from build123d import *

# Parameters (mm, degrees)
BOSS_EXTRUDE1_DEPTH     = 40
CUT_EXTRUDE1_DEPTH      = 60
SKETCH3_W               = 113.025821482
SKETCH3_H               = 33
CUT_EXTRUDE2_DEPTH      = 25
CUT_EXTRUDE6_DEPTH      = 96.088865234
CUT_EXTRUDE6_DEPTH_BACK = 96.088865234
SKETCH7_W               = 50
SKETCH7_H               = 33
SKETCH8_W               = 71.47426929
SKETCH8_H               = 40
BOSS_EXTRUDE2_DEPTH     = 5
FILLET1_R               = 5
FILLET2_R               = 5


with BuildPart() as part:
    # Sketch1 → Boss-Extrude1 (new body)
    with BuildSketch(Plane.XY):
        with BuildLine():
            Line((-56.512910741, 10.211947396), (56.512910741, 10.211947396))
            ThreePointArc((56.512910741, 10.211947396), (82.5, 0), (56.512910741, -10.211947396))
            Line((56.512910741, -10.211947396), (-56.512910741, -10.211947396))
            ThreePointArc((-56.512910741, -10.211947396), (-82.5, 0), (-56.512910741, 10.211947396))
        make_face()
    extrude(amount=BOSS_EXTRUDE1_DEPTH)

    # Sketch2 → Cut-Extrude1 (cut)
    with BuildSketch(Plane.XY.offset(50)):
        with BuildLine():
            Line((44.606109659, 2.95), (-44.606109659, 2.95))
            ThreePointArc((-44.606109659, 2.95), (-47.976180371, 0), (-44.606109659, -2.95))
            Line((-44.606109659, -2.95), (44.606109659, -2.95))
            ThreePointArc((44.606109659, -2.95), (48.007891593, 0), (44.606109659, 2.95))
        make_face()
    extrude(amount=-CUT_EXTRUDE1_DEPTH, mode=Mode.SUBTRACT)

    # Sketch3 → Cut-Extrude2 (cut)
    with BuildSketch(Plane(origin=(0, 10.211947396, 0), x_dir=(1, 0, 0), z_dir=(0, 1, 0))):
        with Locations((0, -20)):
            Rectangle(SKETCH3_W, SKETCH3_H)
    extrude(amount=-CUT_EXTRUDE2_DEPTH, mode=Mode.SUBTRACT)

    # Sketch7 → Cut-Extrude6 (cut, two sides: drawn at the far end of the back side and taken through both)
    with BuildSketch(Plane(origin=(0, 10.211947396, 0), x_dir=(-1, 0, 0), z_dir=(0, -1, 0)).offset(-CUT_EXTRUDE6_DEPTH_BACK)):
        with Locations((81.512910741, -20)):
            Rectangle(SKETCH7_W, SKETCH7_H)
    extrude(amount=CUT_EXTRUDE6_DEPTH + CUT_EXTRUDE6_DEPTH_BACK, mode=Mode.SUBTRACT)

    # Sketch8 → Boss-Extrude2 (add)
    with BuildSketch(Plane(origin=(0, 10.211947396, 0), x_dir=(1, 0, 0), z_dir=(0, 1, 0))):
        with Locations((0, -20)):
            Rectangle(SKETCH8_W, SKETCH8_H)
    extrude(amount=BOSS_EXTRUDE2_DEPTH)

    # Fillet1
    fillet1_edges = [part.edges().sort_by_distance(p)[0] for p in [
        (0, 15.211947396, 40),
    ]]
    fillet(fillet1_edges, radius=FILLET1_R)

    # Fillet2
    fillet2_edges = [part.edges().sort_by_distance(p)[0] for p in [
        (0, 15.211947396, 0),
    ]]
    fillet(fillet2_edges, radius=FILLET2_R)


solid = part.part
Work out the finished part from the listing and answer in its coordinate system (mm). A direction names the side the tool comes from. Give positions to 0.01 mm unless a question says otherwise; leave off trailing zeros. Write each loop counter-clockwise with the first axis right and the second up, starting at its lowest first coordinate (ties: lowest second). Pieces come first, ordered by that corner, then holes. Notation, with made-up numbers: M 48,79 L 68,79 A20 ccw 68,99 Z; hole C 2,46.25 d11. An arc over 180 degrees is marked long. Answer as CSV lines item,"result".
Q1. A cutting plane is placed at D-D on z = 32. Write down the section's boundary in (x, y).
A:
outline,"M -35.74,10.21 L 35.74,10.21 L 35.74,15.21 L -35.74,15.21 Z; M 56.51,-10.21 A15 ccw long 56.51,10.21 Z"
Q2. A cutting plane is placed at A-A on x = 4.5. Write down the section's boundary in (y, z).
A:
outline,"M -10.21,0 L -2.95,0 L -2.95,3.5 L -10.21,3.5 Z; M -10.21,36.5 L -2.95,36.5 L -2.95,40 L -10.21,40 Z; M 2.95,0 L 10.21,0 A5 ccw 15.21,5 L 15.21,35 A5 ccw 10.21,40 L 2.95,40 L 2.95,36.5 L 10.21,36.5 L 10.21,3.5 L 2.95,3.5 Z"
Q3. Find the intervals of material crossed by probe 1 along Y at (x, z) = (-45, 2.15); probe 2 along Z at (x, y) = (-71, 3); probe 3 along Y at (x, z) = (67, 22.5), in increasing order. Write a range as [from, to].
A:
probe 1,"y = [-10.21, -2.98], [2.98, 10.21]"
probe 2,"z = [0, 3.5], [36.5, 40]"
probe 3,"y = [-14.99, 14.99]"
Q4. Given P1, Ø10, axis at y = 1.5, z = 22, coming from the -X side; P2, Ø3, axis at x = 41.5, z = 1.5, coming from the +Y side; P3, Ø1, axis at x = -3.5, z = 1.5, coming from the -Y side, each flat-ended and moving along its own axis, determine where each tip first touches the part or whether it passes through.
A:
P1,"stops at x = 56.51"
P2,"stops at y = 10.21"
P3,"stops at y = -10.21"
Q5. The mould has two halves that part along Z. Classify faces 5 (the flat face through (1, -10.212, 38)), 6 (the flat face through (-14, -3.1, 36.5)), 7 (the cylindrical face through (0.5, 13.786, 1.504)): +Z half, -Z half, draft (parallel to the pull), parting line (faces both ways), or undercut.
A:
face 5,"draft"
face 6,"undercut"
face 7,"-Z half"
Q6. A cutting plane is placed at B-B on y = 0. Write down the section's boundary in (x, z), plus the area to 3 significant figures.
A:
outline,"M -82.5,0 L -47.98,0 L -47.98,3.5 L -82.5,3.5 Z; M -82.5,36.5 L -47.98,36.5 L -47.98,40 L -82.5,40 Z; M 48.01,0 L 82.5,0 L 82.5,40 L 48.01,40 L 48.01,36.5 L 56.51,36.5 L 56.51,3.5 L 48.01,3.5 Z"
area,"1,340 mm²"
Q7. A tool of negligible diameter and unlimited length cuts with its end or side. For faces 1 (the cylindrical face through (48.007, -0.071, 38.274)), 2 (the flat face through (56.513, 0, 20)), 3 (the flat face through (46, 10.212, 2)), 4 (the flat face through (1, -10.212, 2)), from which of +Z, -Z, +X, -X, +Y, -Y can it reach the whole face along a straight path? Write none if from no direction.
A:
face 1,"+Z, -Z"
face 2,"-X, +Y, -Y"
face 3,"+Z, -Z, +Y"
face 4,"+Z, -Z, -Y"
Q8. A cutting plane is placed at C-C on x = -67.5. Write down the section's boundary in (y, z).
A:
outline,"M -15,0 L 15,0 L 15,3.5 L -15,3.5 Z; M -15,36.5 L 15,36.5 L 15,40 L -15,40 Z"
